Check sheet for the modelled part. Datum: model origin and axes. Units: mm. A direction names the side the tool comes from. Give positions to 0.01 mm unless a question says otherwise; leave off trailing zeros. Loops run counter-clockwise (first coordinate to the right, second up) from the corner with the lowest first, then second, coordinate; pieces in that order, holes last. Notation, with made-up numbers: (89, 73.25) -> (102, 73.25) arc R29 cw to (102, 105.25) -> close; hole circle Ø1 at (-6.5, 67). An arc over 180 degrees is marked (long way). Write each question's results on one line, items separated by ' | '. Start each with the question number.
Item 1: Scan lines: line 1 along Y through (x, z) = (0, 0.7); line 2 along Y through (x, z) = (1, 1.5); line 3 along Z through (x, y) = (0, 2.75). Record each from-to range of solid material in increasing order.
Item 2: Cross-section at A-A on y = 0. Enter the section's corners in (x, z).
Item 3: Gauge pin test, flat ends, axial feed: pin 1 Ø1.7 at (x, y) = (-0.5, -1) entering from -Z; pin 2 Ø4 at (y, z) = (-1, 13) entering from +X; pin 3 Ø3 at (x, z) = (-2.5, 15) entering from +Y. Record the tip position at first contact, or that the pin passes through.
Item 4: Access from +Z, -Z, +X, -X, +Y, -Y to the whole of each face (thin tool, end or side, straight path). Record for faces 4 (the face through (3.233, -1.341, 3.451)), 5 (the face through (2.9, 0.1, 1.2)), 6 (the face through (2, -2, 7)).
Item 5: Mould release check, pull along X, two halves, no side actions. Record for faces 1 (the face through (0, 0, 2.5)), 2 (the face through (0, 0, 17)), 3 (the face through (0, -2, 12)): pulls with the +X half, pulls with the -X half, needs draft (parallel to the pull), parting line crosses it, or undercut.
Item 6: Cross-section at D-D on z = 8.25. Enter the section's corners in (x, y), then the cut area to 3 significant figures.
Item 7: Cross-section at B-B on z = 1. Enter the section's corners in (x, y), then the cut area to 3 significant figures.
from build123d import *

# Parameters (mm, degrees)
ESQUISSE1_R             = 3.5
BOSS_EXTRU_1_DEPTH      = 7
ESQUISSE2_R             = 2.9
ENL_V_MAT_EXTRU_1_DEPTH = 2.5
ESQUISSE3_R             = 2
BOSS_EXTRU_2_DEPTH      = 10


with BuildPart() as part:
    # Esquisse1 → Boss.-Extru.1 (new body)
    with BuildSketch(Plane.XY):
        Circle(ESQUISSE1_R)
    extrude(amount=BOSS_EXTRU_1_DEPTH)

    # Esquisse2 → Enlèv. mat.-Extru.1 (cut)
    with BuildSketch(Plane(origin=(0, 0, 0), x_dir=(-1, 0, 0), z_dir=(0, 0, -1))):
        Circle(ESQUISSE2_R)
    extrude(amount=-ENL_V_MAT_EXTRU_1_DEPTH, mode=Mode.SUBTRACT)

    # Esquisse3 → Boss.-Extru.2 (add)
    with BuildSketch(Plane.XY.offset(7)):
        Circle(ESQUISSE3_R)
    extrude(amount=BOSS_EXTRU_2_DEPTH)


solid = part.part
Answer sheet:
1) line 1: y = -3.5 to -2.9, 2.9 to 3.5 | line 2: y = -3.35 to -2.72, 2.72 to 3.35 | line 3: z = 2.5 to 7
2) outline: (-3.5, 0) -> (-2.9, 0) -> (-2.9, 2.5) -> (2.9, 2.5) -> (2.9, 0) -> (3.5, 0) -> (3.5, 7) -> (2, 7) -> (2, 17) -> (-2, 17) -> (-2, 7) -> (-3.5, 7) -> close
3) pin 1: stops at z = 2.5 | pin 2: stops at x = 2 | pin 3: stops at y = 1.73
4) face 4: +Z, -Z | face 5: -Z | face 6: +Z
5) face 1: undercut | face 2: needs draft | face 3: parting line crosses it
6) outline: circle Ø4 at (0, 0) | area: 12.6 mm²
7) outline: circle Ø7 at (0, 0); hole circle Ø5.8 at (0, 0) | area: 12.1 mm²
